from build123d import *

# Parameters (mm, degrees)
SALIENTE_EXTRUIR1_DEPTH      = 5
SALIENTE_EXTRUIR1_DEPTH_BACK = 5
CROQUIS1_W                   = 3
CROQUIS1_H                   = 50
SALIENTE_EXTRUIR3_DEPTH      = 7.5
SALIENTE_EXTRUIR3_DEPTH_BACK = 7.5
CROQUIS1_4_R                 = 3
CROQUIS1_4_R_2               = 1.5
CORTAR_EXTRUIR1_DEPTH        = 2.5
CORTAR_EXTRUIR1_DEPTH_BACK   = 2.5
CROQUIS1_5_R                 = 3
CORTAR_EXTRUIR2_DEPTH        = 10
CORTAR_EXTRUIR2_DEPTH_BACK   = 10
CROQUIS1_6_R                 = 1.5


with BuildPart() as part:
    # Croquis1 → Saliente-Extruir1 (new, two sides: drawn at the far end of the back side and taken through both)
    with BuildSketch(Plane.XY.offset(-SALIENTE_EXTRUIR1_DEPTH_BACK)):
        Rectangle(CROQUIS1_W, CROQUIS1_H)
    extrude(amount=SALIENTE_EXTRUIR1_DEPTH + SALIENTE_EXTRUIR1_DEPTH_BACK)

    # Croquis1<4> → Saliente-Extruir3 (add, two sides: drawn at the far end of the back side and taken through both)
    # profile 1 of 2: a face of its own
    with BuildSketch(Plane.XY.offset(-SALIENTE_EXTRUIR3_DEPTH_BACK)):
        with Locations((0, 25)):
            Circle(CROQUIS1_4_R)
        with Locations((0, 25)):
            Circle(CROQUIS1_4_R_2, mode=Mode.SUBTRACT)
    # profile 2 of 2: a face of its own
    with BuildSketch(Plane.XY.offset(-SALIENTE_EXTRUIR3_DEPTH_BACK)):
        with Locations((0, -25)):
            Circle(CROQUIS1_4_R)
        with Locations((0, -25)):
            Circle(CROQUIS1_4_R_2, mode=Mode.SUBTRACT)
    extrude(amount=SALIENTE_EXTRUIR3_DEPTH + SALIENTE_EXTRUIR3_DEPTH_BACK)

    # Croquis1<5> → Cortar-Extruir1 (cut, two sides: drawn at the far end of the back side and taken through both)
    with BuildSketch(Plane.XY.offset(-CORTAR_EXTRUIR1_DEPTH_BACK)):
        with Locations((0, 25)):
            Circle(CROQUIS1_5_R)
        with Locations((0, -25)):
            Circle(CROQUIS1_5_R)
    extrude(amount=CORTAR_EXTRUIR1_DEPTH + CORTAR_EXTRUIR1_DEPTH_BACK, mode=Mode.SUBTRACT)

    # Croquis1<6> → Cortar-Extruir2 (cut, two sides: drawn at the far end of the back side and taken through both)
    with BuildSketch(Plane.XY.offset(-CORTAR_EXTRUIR2_DEPTH_BACK)):
        with Locations((0, 25)):
            Circle(CROQUIS1_6_R)
        with Locations((0, -25)):
            Circle(CROQUIS1_6_R)
    extrude(amount=CORTAR_EXTRUIR2_DEPTH + CORTAR_EXTRUIR2_DEPTH_BACK, mode=Mode.SUBTRACT)


solid = part.part
Input: part model. Units: mm. Frame: model coordinates. A direction names the side the tool comes from. Coordinates: 2 decimals unless noted, no trailing zeros. Order: outer loops, then holes, each group sorted by start corner. A loop starts at its lowest first (then second) coordinate and runs counter-clockwise, first axis right, second up. Notation, with made-up numbers: M -10,76 L 42,76 A5 cw 42,83 Z; hole C 20.5,84 d2. An arc over 180 degrees is marked long. Answer as CSV lines item,"result".
1. First-contact query: P1, Ø2, axis at x = 1, y = 1.5, coming from the -Z side; P2, Ø3.5, axis at x = -0.5, y = -6, coming from the +Z side; P3, Ø1.8, axis at x = 0, y = -25, coming from the +Z side; P4, Ø1.5, axis at x = -1, z = 4.5, coming from the -Y side. Flat tips, straight axial feed; report the tip coordinate or a pass-through.
Reported:
P1,"z = -5"
P2,"z = 5"
P3,"through"
P4,"y = -27.99"
2. Section C-C (x = 2). Return the cut outline in (y, z).
Reported:
outline,"M -27.24,-7.5 L -22.76,-7.5 L -22.76,-2.5 L -27.24,-2.5 Z; M -27.24,2.5 L -22.76,2.5 L -22.76,7.5 L -27.24,7.5 Z; M 22.76,-7.5 L 27.24,-7.5 L 27.24,-2.5 L 22.76,-2.5 Z; M 22.76,2.5 L 27.24,2.5 L 27.24,7.5 L 22.76,7.5 Z"
3. Pull-direction query (X, two-part tool) for faces 6 (the flat face through (0, 0, 5)), 7 (the flat face through (-1.5, 0, 0)), 8 (the cylindrical face through (0, -22, 0)); classes: released by +X, released by -X, zero draft, split by the parting line, or undercut.
Reported:
face 6,"zero draft"
face 7,"released by -X"
face 8,"undercut"
4. Access query for faces 1 (the cylindrical face through (0, 28, -5)), 2 (the flat face through (1.3, 23.7, -7.5)), 3 (the flat face through (1.5, 0, 0)), 4 (the cylindrical face through (0, 22, 0)), 5 (the flat face through (0, 0, -5)). Directions: +Z, -Z, +X, -X, +Y, -Y. A direction counts if a zero-diameter tool reaches every point of the face in a straight line with its end or side. Return the directions, or none.
Reported:
face 1,"-Z"
face 2,"-Z, +X, -X, +Y, -Y"
face 3,"+Z, -Z, +X"
face 4,"+Y"
face 5,"-Z, +X, -X"
5. Section A-A (y = 25). Return the cut outline in (x, z).
Reported:
outline,"M -3,-7.5 L -1.5,-7.5 L -1.5,-2.5 L -3,-2.5 Z; M -3,2.5 L -1.5,2.5 L -1.5,7.5 L -3,7.5 Z; M 1.5,-7.5 L 3,-7.5 L 3,-2.5 L 1.5,-2.5 Z; M 1.5,2.5 L 3,2.5 L 3,7.5 L 1.5,7.5 Z"
6. Section B-B (z = 6.5). Return the cut outline in (x, y), then the cut area to 3 significant figures.
Reported:
outline,"C 0,-25 d6; C 0,25 d6; hole C 0,-25 d3; hole C 0,25 d3"
area,"42.4 mm2"
7. Material intervals for line 1 (Y direction, x = 0, z = 3.65); line 2 (Y direction, x = 0, z = 6.35); line 3 (Z direction, x = -1.85, y = 24), sorted ascending. Write a range as from..to.
Reported:
line 1,"-28..-26.5, -23.5..23.5, 26.5..28"
line 2,"-28..-26.5, -23.5..-22, 22..23.5, 26.5..28"
line 3,"-7.5..-2.5, 2.5..7.5"
8. Section D-D (z = 3). Return the cut outline in (x, y).
Reported:
outline,"M -1.5,-22.4 A3 ccw long 1.5,-22.4 L 1.5,22.4 A3 ccw long -1.5,22.4 Z; hole C 0,-25 d3; hole C 0,25 d3"
